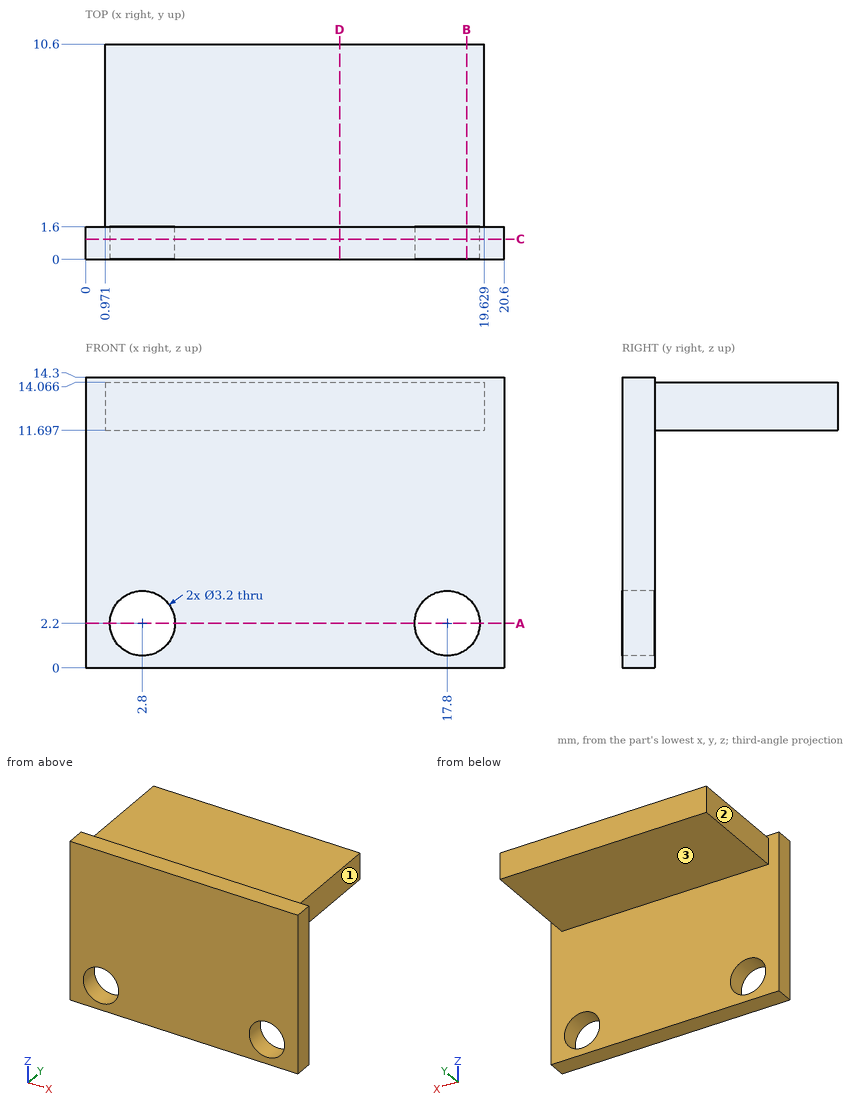
Geometry: see drawing. Coordinates: mm, zero at the bounding-box minimum. A direction names the side the tool comes from. Coordinates: 2 decimals unless noted, no trailing zeros. Order: outer loops, then holes, each group sorted by start corner. A loop starts at its lowest first (then second) coordinate and runs counter-clockwise, first axis right, second up. Notation, with made-up numbers: M 37,61 L 65,61 A22 cw 65,85 Z; hole C 21.25,53 d7. An arc over 180 degrees is marked long. Write each question's results on one line, items separated by ' | '. Start each with the question number.
1) Section query D-D (x = 12.5). Return the cut outline in (y, z).
2) Contact query for flat-ended pins moving along their axis: pin 1 Ø1.9 at (y, z) = (4, 12.5) entering from +X; pin 2 Ø2.5 at (y, z) = (4.5, 12.5) entering from -X; pin 3 Ø4 at (y, z) = (4, 4) entering from -X; pin 4 Ø7 at (x, z) = (5.5, 7.5) entering from +Y. Output: stop coordinate, or through.
3) Line query: line 1 (X direction, y = 0.4, z = 2.2); line 2 (Z direction, x = 2.8, y = 0.3); line 3 (Y direction, x = 19.5, z = 6.5). Output: solid intervals per line, ascending. Write a range as from..to.
4) Section query B-B (x = 18.75). Return the cut outline in (y, z).
5) Section query A-A (z = 2.2). Return the cut outline in (x, y), plus the area to 3 significant figures.
6) Section query C-C (y = 1). Return the cut outline in (x, z), plus the area to 4 significant figures.
7) Access query for the marked faces 1, 2 and 3. Directions: +Z, -Z, +X, -X, +Y, -Y. A direction counts if a zero-diameter tool reaches every point of the face in a straight line with its end or side. Return the directions, or none.
Answers:
1) outline: M 0,0 L 1.6,0 L 1.6,11.7 L 10.6,11.7 L 10.6,14.07 L 1.6,14.07 L 1.6,14.3 L 0,14.3 Z
2) pin 1: stops at x = 19.63 | pin 2: stops at x = 0.97 | pin 3: passes through | pin 4: stops at y = 1.6
3) line 1: x = 0..1.2, 4.4..16.2, 19.4..20.6 | line 2: z = 0..0.6, 3.8..14.3 | line 3: y = 0..1.6
4) outline: M 0,0 L 1.6,0 L 1.6,0.91 L 0,0.91 Z; M 0,3.49 L 1.6,3.49 L 1.6,11.7 L 10.6,11.7 L 10.6,14.07 L 1.6,14.07 L 1.6,14.3 L 0,14.3 Z
5) outline: M 0,0 L 1.2,0 L 1.2,1.6 L 0,1.6 Z; M 4.4,0 L 16.2,0 L 16.2,1.6 L 4.4,1.6 Z; M 19.4,0 L 20.6,0 L 20.6,1.6 L 19.4,1.6 Z | area: 22.7 mm^2
6) outline: M 0,0 L 20.6,0 L 20.6,14.3 L 0,14.3 Z; hole C 2.8,2.2 d3.2; hole C 17.8,2.2 d3.2 | area: 278.5 mm^2
7) face 1: +Z, -Z, +X, +Y | face 2: +Z, -Z, -X, +Y | face 3: -Z, +X, -X, +Y
